Check sheet for the modelled part. Datum: model origin and axes. Units: mm. Round coordinates to 2 decimals unless told otherwise and drop trailing zeros. Order: outer loops, then holes, each group sorted by start corner. A loop starts at its lowest first (then second) coordinate and runs counter-clockwise, first axis right, second up. Notation, with made-up numbers: (82.5, 60.25) -> (124.5, 60.25) arc R3 ccw to (124.5, 64.25) -> close; hole circle Ø3 at (-6, 5). An arc over 180 degrees is marked (long way). Answer as CSV lines item,"result". Start each with the question number.
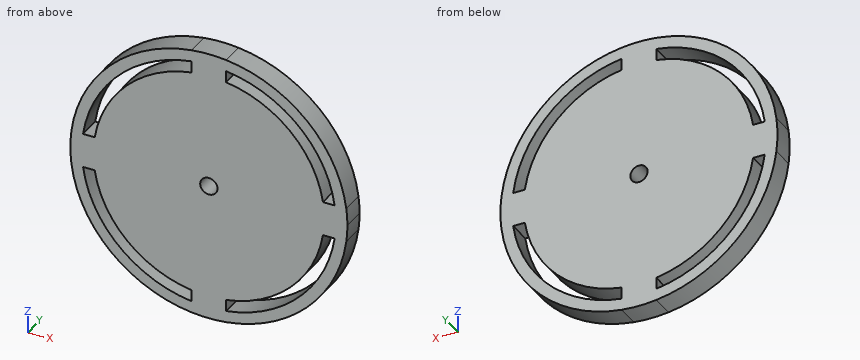
from build123d import *

# Parameters (mm, degrees)
F0_W     = 19.05
F0_H     = 19.05
F0_R     = 4.7625
F1_DEPTH = 12.7


with BuildPart() as f1:
    # F0 (on Front) → F1 (new body)
    with BuildSketch(Plane.XZ):
        with BuildLine():
            ThreePointArc((75.6023437137, -9.525), (76.0504391538, -4.7718659358), (76.2, 0))
            ThreePointArc((76.2, 0), (76.0504391538, 4.7718659358), (75.6023437137, 9.525))
            Line((75.6023437137, 9.525), (69.1975207287, 9.525))
            ThreePointArc((69.1975207287, 9.525), (69.6866892703, 4.7736609169), (69.85, 0))
            ThreePointArc((69.85, 0), (69.6866892703, -4.7736609169), (69.1975207287, -9.525))
            Line((69.1975207287, -9.525), (75.6023437137, -9.525))
        make_face()
        with BuildLine():
            Line((69.1975207287, 9.525), (75.6023437137, 9.525))
            ThreePointArc((75.6023437137, 9.525), (53.8815367264, 53.8815367264), (9.525, 75.6023437137))
            Line((9.525, 75.6023437137), (9.525, 69.1975207287))
            ThreePointArc((9.525, 69.1975207287), (49.3914086659, 49.3914086659), (69.1975207287, 9.525))
        make_face()
        with BuildLine():
            ThreePointArc((9.525, -75.6023437137), (53.8815367264, -53.8815367264), (75.6023437137, -9.525))
            Line((75.6023437137, -9.525), (69.1975207287, -9.525))
            ThreePointArc((69.1975207287, -9.525), (49.3914086659, -49.3914086659), (9.525, -69.1975207287))
            Line((9.525, -69.1975207287), (9.525, -75.6023437137))
        make_face()
        with BuildLine():
            Line((9.525, 69.1975207287), (9.525, 75.6023437137))
            ThreePointArc((9.525, 75.6023437137), (0, 76.2), (-9.525, 75.6023437137))
            Line((-9.525, 75.6023437137), (-9.525, 69.1975207287))
            ThreePointArc((-9.525, 69.1975207287), (0, 69.85), (9.525, 69.1975207287))
        make_face()
        with BuildLine():
            ThreePointArc((-9.525, -75.6023437137), (0, -76.2), (9.525, -75.6023437137))
            Line((9.525, -75.6023437137), (9.525, -69.1975207287))
            ThreePointArc((9.525, -69.1975207287), (0, -69.85), (-9.525, -69.1975207287))
            Line((-9.525, -69.1975207287), (-9.525, -75.6023437137))
        make_face()
        with BuildLine():
            Line((-9.525, 69.1975207287), (-9.525, 75.6023437137))
            ThreePointArc((-9.525, 75.6023437137), (-53.8815367264, 53.8815367264), (-75.6023437137, 9.525))
            Line((-75.6023437137, 9.525), (-69.1975207287, 9.525))
            ThreePointArc((-69.1975207287, 9.525), (-49.3914086659, 49.3914086659), (-9.525, 69.1975207287))
        make_face()
        with BuildLine():
            ThreePointArc((-75.6023437137, -9.525), (-53.8815367264, -53.8815367264), (-9.525, -75.6023437137))
            Line((-9.525, -75.6023437137), (-9.525, -69.1975207287))
            ThreePointArc((-9.525, -69.1975207287), (-49.3914086659, -49.3914086659), (-69.1975207287, -9.525))
            Line((-69.1975207287, -9.525), (-75.6023437137, -9.525))
        make_face()
        with BuildLine():
            Line((-69.1975207287, 9.525), (-75.6023437137, 9.525))
            ThreePointArc((-75.6023437137, 9.525), (-76.2, 0), (-75.6023437137, -9.525))
            Line((-75.6023437137, -9.525), (-69.1975207287, -9.525))
            ThreePointArc((-69.1975207287, -9.525), (-69.85, 0), (-69.1975207287, 9.525))
        make_face()
        with BuildLine():
            Line((-9.525, 9.525), (-9.525, 62.7815607882))
            ThreePointArc((-9.525, 62.7815607882), (-44.9012806053, 44.9012806053), (-62.7815607882, 9.525))
            Line((-62.7815607882, 9.525), (-9.525, 9.525))
        make_face()
        with BuildLine():
            Line((9.525, 9.525), (62.7815607882, 9.525))
            ThreePointArc((62.7815607882, 9.525), (44.9012806053, 44.9012806053), (9.525, 62.7815607882))
            Line((9.525, 62.7815607882), (9.525, 9.525))
        make_face()
        with BuildLine():
            ThreePointArc((9.525, -62.7815607882), (44.9012806053, -44.9012806053), (62.7815607882, -9.525))
            Line((62.7815607882, -9.525), (9.525, -9.525))
            Line((9.525, -9.525), (9.525, -62.7815607882))
        make_face()
        with BuildLine():
            ThreePointArc((-62.7815607882, -9.525), (-44.9012806053, -44.9012806053), (-9.525, -62.7815607882))
            Line((-9.525, -62.7815607882), (-9.525, -9.525))
            Line((-9.525, -9.525), (-62.7815607882, -9.525))
        make_face()
        with BuildLine():
            Line((-9.525, -9.525), (-9.525, 9.525))
            Line((-9.525, 9.525), (-62.7815607882, 9.525))
            ThreePointArc((-62.7815607882, 9.525), (-63.5, 0), (-62.7815607882, -9.525))
            Line((-62.7815607882, -9.525), (-9.525, -9.525))
        make_face()
        with BuildLine():
            ThreePointArc((63.5, 0), (63.3201354628, 4.776028159), (62.7815607882, 9.525))
            Line((62.7815607882, 9.525), (9.525, 9.525))
            Line((9.525, 9.525), (9.525, -9.525))
            Line((9.525, -9.525), (62.7815607882, -9.525))
            ThreePointArc((62.7815607882, -9.525), (63.3201354628, -4.776028159), (63.5, 0))
        make_face()
        with BuildLine():
            Line((9.525, 9.525), (9.525, 62.7815607882))
            ThreePointArc((9.525, 62.7815607882), (0, 63.5), (-9.525, 62.7815607882))
            Line((-9.525, 62.7815607882), (-9.525, 9.525))
            Line((-9.525, 9.525), (9.525, 9.525))
        make_face()
        with BuildLine():
            ThreePointArc((-9.525, -62.7815607882), (0, -63.5), (9.525, -62.7815607882))
            Line((9.525, -62.7815607882), (9.525, -9.525))
            Line((9.525, -9.525), (-9.525, -9.525))
            Line((-9.525, -9.525), (-9.525, -62.7815607882))
        make_face()
        Rectangle(F0_W, F0_H)
        Circle(F0_R, mode=Mode.SUBTRACT)
        with BuildLine():
            Line((9.525, 62.7815607882), (9.525, 69.1975207287))
            ThreePointArc((9.525, 69.1975207287), (0, 69.85), (-9.525, 69.1975207287))
            Line((-9.525, 69.1975207287), (-9.525, 62.7815607882))
            ThreePointArc((-9.525, 62.7815607882), (0, 63.5), (9.525, 62.7815607882))
        make_face()
        with BuildLine():
            Line((-62.7815607882, 9.525), (-69.1975207287, 9.525))
            ThreePointArc((-69.1975207287, 9.525), (-69.85, 0), (-69.1975207287, -9.525))
            Line((-69.1975207287, -9.525), (-62.7815607882, -9.525))
            ThreePointArc((-62.7815607882, -9.525), (-63.5, 0), (-62.7815607882, 9.525))
        make_face()
        with BuildLine():
            ThreePointArc((-9.525, -69.1975207287), (0, -69.85), (9.525, -69.1975207287))
            Line((9.525, -69.1975207287), (9.525, -62.7815607882))
            ThreePointArc((9.525, -62.7815607882), (0, -63.5), (-9.525, -62.7815607882))
            Line((-9.525, -62.7815607882), (-9.525, -69.1975207287))
        make_face()
        with BuildLine():
            ThreePointArc((69.85, 0), (69.6866892703, 4.7736609169), (69.1975207287, 9.525))
            Line((69.1975207287, 9.525), (62.7815607882, 9.525))
            ThreePointArc((62.7815607882, 9.525), (63.3201354628, 4.776028159), (63.5, 0))
            ThreePointArc((63.5, 0), (63.3201354628, -4.776028159), (62.7815607882, -9.525))
            Line((62.7815607882, -9.525), (69.1975207287, -9.525))
            ThreePointArc((69.1975207287, -9.525), (69.6866892703, -4.7736609169), (69.85, 0))
        make_face()
    extrude(amount=F1_DEPTH)


solid = f1.part
1) Depth check by flat-ended pin: pin 1 Ø2 at (x, y) = (24.5, -3.5) entering from -Z; pin 2 Ø6 at (x, y) = (-10.5, -7) entering from +Z; pin 3 Ø1 at (y, z) = (-11, 47.5) entering from -X. Enter the tip coordinate at first touch or a pass-through.
2) Section check D-D on y = -3.25. Count the separate pieces of the cut face and the enclosed holes in it, then the cut area to 3 significant figures.
3) Section check C-C on x = 52. Record the cut outline in (y, z), then the cut area to 3 significant figures.
4) Section check B-B on z = -34.5. Record the cut outline in (x, y), then the cut area to 3 significant figures.
5) Section check A-A on x = 0. Record the cut outline in (y, z), then the cut area to 3 significant figures.
6) Material ranges on line 1 along Z through (x, y) = (0, -7); line 2 along Z through (x, y) = (-16, -2.75); line 3 along Z through (x, y) = (-29, -5), recorded low to high.
Solutions:
1,pin 1,"stops at z = -72.49"
1,pin 2,"stops at z = 75.83"
1,pin 3,"stops at x = -59.98"
2,separate pieces,"1"
2,enclosed holes,"5"
2,area,"16,000 mm^2"
3,outline,"(-12.7, -55.7) -> (0, -55.7) -> (0, -46.64) -> (-12.7, -46.64) -> close; (-12.7, -36.45) -> (0, -36.45) -> (0, 36.45) -> (-12.7, 36.45) -> close; (-12.7, 46.64) -> (0, 46.64) -> (0, 55.7) -> (-12.7, 55.7) -> close"
3,area,"1,160 mm^2"
4,outline,"(-67.94, -12.7) -> (-60.74, -12.7) -> (-60.74, 0) -> (-67.94, 0) -> close; (-53.31, -12.7) -> (53.31, -12.7) -> (53.31, 0) -> (-53.31, 0) -> close; (60.74, -12.7) -> (67.94, -12.7) -> (67.94, 0) -> (60.74, 0) -> close"
4,area,"1,540 mm^2"
5,outline,"(-12.7, -76.2) -> (0, -76.2) -> (0, -4.76) -> (-12.7, -4.76) -> close; (-12.7, 4.76) -> (0, 4.76) -> (0, 76.2) -> (-12.7, 76.2) -> close"
5,area,"1,810 mm^2"
6,line 1,"z = -76.2 to -4.76, 4.76 to 76.2"
6,line 2,"z = -74.5 to -67.99, -61.45 to 61.45, 67.99 to 74.5"
6,line 3,"z = -70.47 to -63.55, -56.49 to 56.49, 63.55 to 70.47"
